from build123d import *

# Parameters (mm, degrees)
EXTRUDE_1_DEPTH     = 1
SKETCH_3_R          = 2.952738467
SKETCH_5_R          = 1.738152606
SKETCH_6_W          = 0.733255876
SKETCH_6_H          = 1.533688363
EXTRUDE_2_DEPTH     = 2.4
CUT_EXTRUDE_1_DEPTH = 2.4
FILLET_1_R          = 0.2
FILLET_2_R          = 0.2
SKETCH_8_R          = 1.529357016
CUT_EXTRUDE_3_DEPTH = 0.2


with BuildPart() as part:
    # 草图2 → 凸台-拉伸1 (new body)
    with BuildSketch(Plane.XY):
        with BuildLine():
            Line((20.507695312, 136.955018135), (22.681412951, 146.041906443))
            ThreePointArc((22.681412951, 146.041906443), (24.498369442, 147.476769267), (26.317825582, 146.045077413))
            Line((26.317825582, 146.045077413), (28.492304397, 136.955019349))
            ThreePointArc((28.492304397, 136.955019349), (24.500000624, 131.895057082), (20.507695312, 136.955018135))
        make_face()
    extrude_1 = extrude(amount=EXTRUDE_1_DEPTH)

    # 草图3 → 放样2 section 0
    with BuildSketch(Plane.XY.offset(1)):
        with Locations((24.5, 136)):
            Circle(SKETCH_3_R)
    # 草图5 → 放样2 section 1
    with BuildSketch(Plane(origin=(0, 0, 2.2), x_dir=(-1, 0, 0), z_dir=(0, 0, -1))):
        with Locations((-24.5, 136)):
            Circle(SKETCH_5_R)
    loft_2 = loft()

    # 草图6 → 凸台-拉伸2 (add)
    with BuildSketch(Plane.XY.offset(1)):
        with Locations((24.5, 145.257576629)):
            Rectangle(SKETCH_6_W, SKETCH_6_H)
    extrude(amount=EXTRUDE_2_DEPTH)

    # 草图7 → 切除-拉伸1 (cut)
    with BuildSketch(Plane.ZY.offset(-24.133372062)):
        Polygon((1.884714406, 146.02442081), (3.4, 144.490732447), (3.4, 146.02442081), align=None)
    extrude(amount=-CUT_EXTRUDE_1_DEPTH, mode=Mode.SUBTRACT)

    # 圆角1
    fillet_1_edges = [part.edges().sort_by_distance(p)[0] for p in [
        (24.5, 144.490732447, 3.4),
        (24.5, 146.02442081, 1.884714406),
    ]]
    fillet(fillet_1_edges, radius=FILLET_1_R)

    # 镜向4: 放样2 across plane
    add(loft_2.mirror(Plane(origin=(0, 0, 2.2), x_dir=(1, 0, 0), z_dir=(0, 0, -1))))

    # 镜向5: 凸台-拉伸1 across plane
    add(extrude_1.mirror(Plane(origin=(0, 0, 2.2), x_dir=(1, 0, 0), z_dir=(0, 0, -1))))

    # 圆角2
    fillet_2_edges = [part.edges().sort_by_distance(p)[0] for p in [
        (22.761847394, 136, 2.2),
    ]]
    fillet(fillet_2_edges, radius=FILLET_2_R)

    # 草图8 → 切除-拉伸3 (cut)
    with BuildSketch(Plane.XY.offset(4.4)):
        with Locations((24.5, 136)):
            Circle(SKETCH_8_R)
    extrude(amount=-CUT_EXTRUDE_3_DEPTH, mode=Mode.SUBTRACT)


solid = part.part
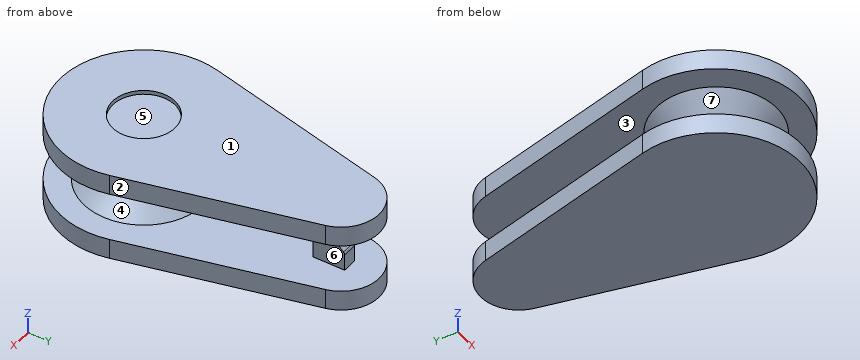
Can you work these out from the model? Positions are in its coordinate system, mm. Face numbers are marked on the shaded views. A direction names the side the tool comes from. Coordinates: 2 decimals unless noted, no trailing zeros. Loops run counter-clockwise (first coordinate to the right, second up) from the corner with the lowest first, then second, coordinate; pieces in that order, holes last. Notation, with made-up numbers: (67.5, -22.5) - (126.5, -22.5) arc R18 ccw to (126.5, 10.5) - close; hole circle Ø3 at (15.5, -13.5). An arc over 180 degrees is marked (long way). Answer as a JSON object with one key per item and string values. Group by question number.
Item 1: If we section it at B-B (z = 3.9): List the corners of the cut face in (x, y) for me, plus the area to 3 significant figures.
Item 2: On a 3-axis mill with a long thin cutter (end or side, diameter ignored), from which of +Z, -Z, +X, -X, +Y, -Y can I reach the whole of each face in a straight line? I mean the marked faces 5, 6 and 7. Say none if no direction works.
Item 3: If we section it at A-A (y = 142.75): List the corners of the cut face in (x, z) for me, plus the area to 3 significant figures.
Item 4: If we mould it in two halves opening along Z, with no side actions, what happens to the marked faces 1, 2, 3 and 4? For each: released by +Z, released by -Z, zero draft, split by the parting line, or undercut.
Item 5: For pin 1 (0.8 mm diameter, centred on x = 24.5, z = 1.5, fed in from +Y); pin 2 (0.5 mm diameter, centred on y = 145.5, z = 2, fed in from -X); pin 3 (1.5 mm diameter, centred on x = 25, y = 136, fed in from +Z); pin 4 (1.5 mm diameter, centred on y = 143, z = 2, fed in from -X), each with a flat end and sliding along its axis, tell me the tip position at first contact or that it passes through.
Item 6: If I drill on L1, parallel to Z at x = 27.25, y = 134; L2, parallel to Y at x = 24.5, z = 4.35; L3, parallel to X at y = 136, z = 4.25, over which ranges is the centre line in solid material (lowest first)? Write a range as from..to.
Item 7: If we section it at C-C (y = 145): List the corners of the cut face in (x, z) for me.
Returned:
{
 "1": {"outline": "(20.51, 136.96) arc R4.1 ccw (long way) to (28.49, 136.96) - (26.32, 146.05) arc R1.87 ccw to (22.68, 146.04) - close", "area": "90.9 mm²"},
 "2": {"face 5": "+Z", "face 6": "+X, +Y", "face 7": "none"},
 "3": {"outline": "(21.89, 0) - (27.11, 0) - (27.11, 1) - (21.89, 1) - close; (21.89, 3.4) - (27.11, 3.4) - (27.11, 4.4) - (21.89, 4.4) - close", "area": "10.4 mm²"},
 "4": {"face 1": "released by +Z", "face 2": "zero draft", "face 3": "undercut", "face 4": "undercut"},
 "5": {"pin 1": "stops at y = 146.02", "pin 2": "stops at x = 24.13", "pin 3": "stops at z = 4.2", "pin 4": "passes through"},
 "6": {"L1": "z = 0..1, 3.4..4.4", "L2": "y = 131.9..134.47, 137.53..147.48", "L3": "x = 20.4..22.97, 26.03..28.6"},
 "7": {"outline": "(22.43, 0) - (26.57, 0) - (26.57, 1) - (24.87, 1) - (24.87, 2.9) - (24.13, 2.9) - (24.13, 1) - (22.43, 1) - close; (22.43, 3.4) - (26.57, 3.4) - (26.57, 4.4) - (22.43, 4.4) - close"}
}
